Source: CAD feature listing. Evaluate the final solid. Frame: model axes, mm. A direction names the side the tool comes from. Give positions to 0.01 mm unless a question says otherwise; leave off trailing zeros. Order: outer loops, then holes, each group sorted by start corner. A loop starts at its lowest first (then second) coordinate and runs counter-clockwise, first axis right, second up. Notation, with made-up numbers: (14.5, 71) -> (23.5, 71) arc R23 ccw to (23.5, 95) -> close; hole circle Ø8 at (51.25, -29). An arc over 180 degrees is marked (long way). Answer in a Markdown table with one row per item.
```python
from build123d import *

# Parameters (mm, degrees)
SKETCH1_W           = 45
SKETCH1_H           = 30
SKETCH1_R           = 1.7
SKETCH1_W_2         = 24
SKETCH1_H_2         = 43.058371989
SKETCH1_R_2         = 2.2
BOSS_EXTRUDE2_DEPTH = 17
SKETCH5_W           = 12
SKETCH5_H           = 100
CUT_EXTRUDE1_DEPTH  = 8
SKETCH7_W           = 29.697028674
SKETCH7_H           = 34.988499238
CUT_EXTRUDE2_DEPTH  = 7
SKETCH9_W           = 45
SKETCH9_H           = 30
BOSS_EXTRUDE3_DEPTH = 10
FILLET1_R           = 7
FILLET6_R           = 2
FILLET7_R           = 1
FILLET8_R           = 4


with BuildPart() as part:
    # Sketch1 → Boss-Extrude2 (new body)
    with BuildSketch(Plane(origin=(0, 0, 0), x_dir=(1, 0, 0), z_dir=(0, 1, 0))):
        Rectangle(SKETCH1_W, SKETCH1_H)
        with Locations((-10, 10)):
            Circle(SKETCH1_R, mode=Mode.SUBTRACT)
        with Locations((10, 10)):
            Circle(SKETCH1_R, mode=Mode.SUBTRACT)
        with Locations((10, -10)):
            Circle(SKETCH1_R, mode=Mode.SUBTRACT)
        with Locations((-10, -10)):
            Circle(SKETCH1_R, mode=Mode.SUBTRACT)
        with Locations((0, -36.529185995)):
            Rectangle(SKETCH1_W_2, SKETCH1_H_2)
        with Locations((0, -25)):
            Circle(SKETCH1_R_2, mode=Mode.SUBTRACT)
        with Locations((0, -50)):
            Circle(SKETCH1_R_2, mode=Mode.SUBTRACT)
    extrude(amount=-BOSS_EXTRUDE2_DEPTH)

    # Sketch5 → Cut-Extrude1 (cut)
    with BuildSketch(Plane(origin=(0, 0, 0), x_dir=(1, 0, 0), z_dir=(0, 1, 0))):
        with Locations((0, -16.465194583)):
            Rectangle(SKETCH5_W, SKETCH5_H)
    extrude(amount=-CUT_EXTRUDE1_DEPTH, mode=Mode.SUBTRACT)

    # Sketch7 → Cut-Extrude2 (cut, through all)
    with BuildSketch(Plane(origin=(0, -6, 0), x_dir=(1, 0, 0), z_dir=(0, 1, 0))):
        with Locations((-0.809918964, -42.047133079)):
            Rectangle(SKETCH7_W, SKETCH7_H)
    extrude(amount=CUT_EXTRUDE2_DEPTH, mode=Mode.SUBTRACT)

    # Sketch9 → Boss-Extrude3 (add)
    with BuildSketch(Plane.XZ.offset(17)):
        Rectangle(SKETCH9_W, SKETCH9_H)
    extrude(amount=BOSS_EXTRUDE3_DEPTH)

    # Fillet1
    fillet1_edges = [part.edges().sort_by_distance(p)[0] for p in [
        (-12, -8.5, 15),
        (12, -8.5, 15),
    ]]
    fillet(fillet1_edges, radius=FILLET1_R)

    # Fillet6
    fillet6_edges = [part.edges().sort_by_distance(p)[0] for p in [
        (22.5, -13.5, 15),
        (-22.5, -13.5, 15),
        (-22.5, -13.5, -15),
        (22.5, -13.5, -15),
        (9, -6, 24.55288346),
        (-9, -6, 24.55288346),
    ]]
    fillet(fillet6_edges, radius=FILLET6_R)

    # Fillet7
    fillet7_edges = [part.edges().sort_by_distance(p)[0] for p in [
        (-12, -2, 24.55288346),
        (12, -2, 24.55288346),
        (-12, -5.414213562, 25.138669897),
        (12, -5.414213562, 25.138669897),
        (-12, -11.5, 58.058371989),
        (12, -11.5, 58.058371989),
        (0, -17, 58.058371989),
        (9, 0, 24.55288346),
        (9, -6, 58.058371989),
        (12, -6, 42.305627724),
        (-9, 0, 24.55288346),
        (-9, -6, 58.058371989),
        (-12, -6, 42.305627724),
    ]]
    fillet(fillet7_edges, radius=FILLET7_R)

    # Fillet8
    fillet8_edges = [part.edges().sort_by_distance(p)[0] for p in [
        (0, -17, 15),
    ]]
    fillet(fillet8_edges, radius=FILLET8_R)


solid = part.part
```
(1) Section query D-D (z = -4). Return the cut outline in (x, y).
A:
| item | result |
|---|---|
| outline | (-22.5, -27) -> (22.5, -27) -> (22.5, 0) -> (6, 0) -> (6, -8) -> (-6, -8) -> (-6, 0) -> (-22.5, 0) -> close |
(2) Section query A-A (z = 50). Return the cut outline in (x, y), plus the area to 3 significant figures.
A:
| item | result |
|---|---|
| outline | (-12, -17) -> (-2.2, -17) -> (-2.2, -8) -> (-6, -8) -> (-6, -6) -> (-11, -6) arc R1 ccw to (-12, -7) -> close; (2.2, -17) -> (12, -17) -> (12, -7) arc R1 ccw to (11, -6) -> (6, -6) -> (6, -8) -> (2.2, -8) -> close |
| area | 200 mm^2 |
(3) First-contact query: pin 1 Ø8.5 at (y, z) = (-8, 36.5) entering from +X; pin 2 Ø1.5 at (x, z) = (-9.5, 33.5) entering from -Y; pin 3 Ø3.5 at (x, y) = (-7.5, -3) entering from +Z; pin 4 Ø3.5 at (x, z) = (0, 25) entering from -Y. Flat tips, straight axial feed; report the tip coordinate or a pass-through.
A:
| item | result |
|---|---|
| pin 1 | stops at x = 12 |
| pin 2 | stops at y = -17 |
| pin 3 | stops at z = 24.7 |
| pin 4 | passes through |
(4) Access query for faces 5 (the flat face through (-12, -12, 40)), 6 (the flat face through (0, -17, 38)), 7 (the flat face through (-6, -5, 14)). Directions: +Z, -Z, +X, -X, +Y, -Y. A direction counts if a zero-diameter tool reaches every point of the face in a straight line with its end or side. Return the directions, or none.
A:
| item | result |
|---|---|
| face 5 | +Z, -X, +Y, -Y |
| face 6 | +Z, +X, -X, -Y |
| face 7 | +Z, -Z, +Y |
(5) Pull-direction query (Z, two-part tool) for faces 1 (the cylindrical face through (-14, -8.3, 17.1)), 2 (the cylindrical face through (9.63, -8.38, 11.66)), 3 (the cylindrical face through (9.63, -8.38, -8.34)), 4 (the flat face through (-22.5, -13, 0)); classes: +Z half, -Z half, draft (parallel to the pull), parting line (faces both ways), or undercut.
A:
| item | result |
|---|---|
| face 1 | +Z half |
| face 2 | undercut |
| face 3 | undercut |
| face 4 | draft |
(6) Section query B-B (y = -10.5). Return the cut outline in (x, z), plus the area to 3 significant figures.
A:
| item | result |
|---|---|
| outline | (-22.5, -13) arc R2 ccw to (-20.5, -15) -> (20.5, -15) arc R2 ccw to (22.5, -13) -> (22.5, 13) arc R2 ccw to (20.5, 15) -> (19, 15) arc R7 cw to (12, 22) -> (12, 57.06) arc R1 ccw to (11, 58.06) -> (-11, 58.06) arc R1 ccw to (-12, 57.06) -> (-12, 22) arc R7 cw to (-19, 15) -> (-20.5, 15) arc R2 ccw to (-22.5, 13) -> close; hole circle Ø3.4 at (-10, -10); hole circle Ø3.4 at (-10, 10); hole circle Ø4.4 at (0, 25); hole circle Ø4.4 at (0, 50); hole circle Ø3.4 at (10, -10); hole circle Ø3.4 at (10, 10) |
| area | 2,330 mm^2 |
(7) Section query C-C (x = 3). Return the cut outline in (y, z), plus the area to 3 significant figures.
A:
| item | result |
|---|---|
| outline | (-27, -15) -> (-8, -15) -> (-8, 58.06) -> (-16, 58.06) arc R1 ccw to (-17, 57.06) -> (-17, 19) arc R4 cw to (-21, 15) -> (-27, 15) -> close |
| area | 961 mm^2 |
(8) Ray query, probe 1 along X at (y, z) = (-9.75, 10); probe 2 along Z at (x, y) = (0, -13.75); probe 3 along X at (y, z) = (-4.5, 10). Return the intervals inside material, ascending.
A:
| item | result |
|---|---|
| probe 1 | x = -22.5 to -11.7, -8.3 to 8.3, 11.7 to 22.5 |
| probe 2 | z = -15 to 22.8, 27.2 to 47.8, 52.2 to 58.06 |
| probe 3 | x = -22.5 to -11.7, -8.3 to -6, 6 to 8.3, 11.7 to 22.5 |
